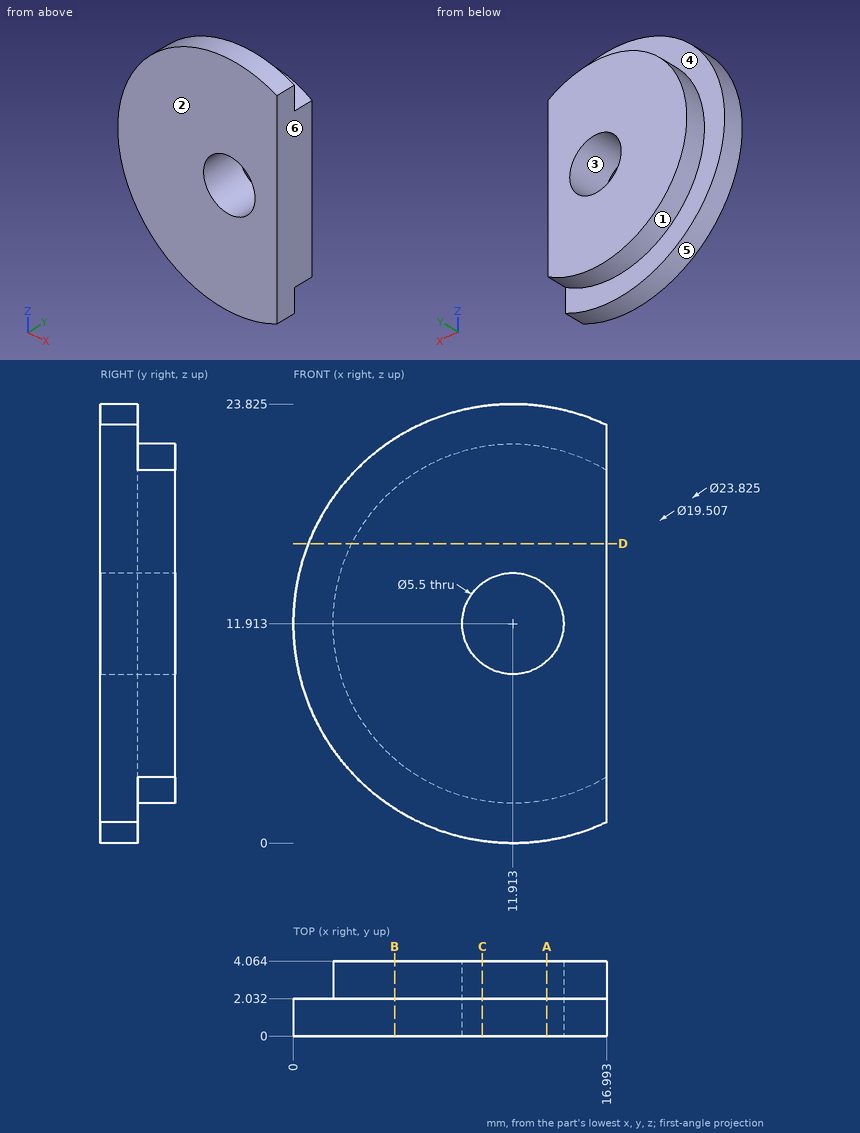
Can you work these out from the drawing? Everything is in mm from the part's minimum corner. A direction names the side the tool comes from. Give positions to 0.01 mm unless a question says otherwise; leave off trailing zeros. Loops run counter-clockwise (first coordinate to the right, second up) from the corner with the lowest first, then second, coordinate; pieces in that order, holes last. Notation, with made-up numbers: (59, 3.25) -> (75, 3.25) arc R24 ccw to (75, 25.25) -> close; hole circle Ø3 at (23.25, 41). An arc over 180 degrees is marked (long way). Return JSON: item names as keys, results as strings.
Item 1: If we section it at C-C on x = 10.25: List the corners of the cut face in (y, z) for me.
Geometry results:
{"outline": "(0, 0.12) -> (2.03, 0.12) -> (2.03, 2.3) -> (4.06, 2.3) -> (4.06, 9.72) -> (0, 9.72) -> close; (0, 14.1) -> (4.06, 14.1) -> (4.06, 21.52) -> (2.03, 21.52) -> (2.03, 23.71) -> (0, 23.71) -> close"}
Item 2: If we section it at D-D on z = 16.25: List the corners of the cut face in (x, y) for me.
Geometry results:
{"outline": "(0.82, 0) -> (16.99, 0) -> (16.99, 4.06) -> (3.18, 4.06) -> (3.18, 2.03) -> (0.82, 2.03) -> close"}
Item 3: If we section it at B-B on x = 5.5: List the corners of the cut face in (y, z) for me.
Geometry results:
{"outline": "(0, 1.87) -> (2.03, 1.87) -> (2.03, 4.56) -> (4.06, 4.56) -> (4.06, 19.26) -> (2.03, 19.26) -> (2.03, 21.95) -> (0, 21.95) -> close"}
Item 4: We'd pull the mould along X, two halves only. Please class the marked faces 3, 4, 5 and 6: +X half, -X half, draft (parallel to the pull), parting line (faces both ways), or undercut.
Geometry results:
{"face 3": "undercut", "face 4": "draft", "face 5": "parting line", "face 6": "+X half"}
Item 5: Which directions (+Z, -Z, +X, -X, +Y, -Y) give clear straight access to the entire face, cutting with the end or side of a thin tool? Please do the marked faces 1 and 2.
Geometry results:
{"face 1": "+Y", "face 2": "+Z, -Z, +X, -X, -Y"}
Item 6: If we section it at A-A on x = 13.75: List the corners of the cut face in (y, z) for me.
Geometry results:
{"outline": "(0, 0.14) -> (2.03, 0.14) -> (2.03, 2.33) -> (4.06, 2.33) -> (4.06, 9.87) -> (0, 9.87) -> close; (0, 13.96) -> (4.06, 13.96) -> (4.06, 21.49) -> (2.03, 21.49) -> (2.03, 23.68) -> (0, 23.68) -> close"}
Item 7: I need wall thicknesses on L1, parallel to Z at x = 12, y = 1.05 (1 decimal); L2, parallel to X at y = 1.25, z = 18.75; L3, parallel to X at y = 2.55, z = 11. Which ranges of each line are inside material? Lowest first, please. Write a range as from..to.
Geometry results:
{"L1": "z = 0..9.2, 14.7..23.8", "L2": "x = 2.16..16.99", "L3": "x = 2.2..9.32, 14.51..16.99"}
